from build123d import *

# Parameters (mm, degrees)
F1_DEPTH = 3
F2_DEPTH = 150
F3_R     = 30.5
F3_R_2   = 1
F4_DEPTH = 5
F5_R     = 30.5
F5_R_2   = 1
F6_DEPTH = 5


with BuildPart() as f1:
    # F0 (on Top) → F1 (new body)
    with BuildSketch(Plane.XY):
        Polygon((-91.6025403784, 38.2228657698), (-91.6025403784, -34.6638855762), (-1.3397459622, -86.7771342302), (105, -86.7771342302), (105, 38.2228657698), align=None)
        Polygon((100, -81.7771342302), (0, -81.7771342302), (-86.6025403784, -31.7771342302), (-86.6025403784, 33.2228657698), (100, 33.2228657698), align=None, mode=Mode.SUBTRACT)
        Polygon((-86.6025403784, -31.7771342302), (0, -81.7771342302), (100, -81.7771342302), (100, 33.2228657698), (-86.6025403784, 33.2228657698), align=None)
    extrude(amount=F1_DEPTH)

    # F0 (on Top) → F2 (join)
    with BuildSketch(Plane.XY):
        Polygon((-91.6025403784, 38.2228657698), (-91.6025403784, -34.6638855762), (-1.3397459622, -86.7771342302), (105, -86.7771342302), (105, 38.2228657698), align=None)
        Polygon((100, -81.7771342302), (0, -81.7771342302), (-86.6025403784, -31.7771342302), (-86.6025403784, 33.2228657698), (100, 33.2228657698), align=None, mode=Mode.SUBTRACT)
    extrude(amount=F2_DEPTH)

    # F3 (on face) → F4 (cut)
    with BuildSketch(Plane.XZ.offset(86.7771342302)):
        with Locations((51.8301270189, 39.6802276373)):
            Circle(F3_R)
        with Locations((25.3301270189, 13.1802276373)):
            Circle(F3_R_2)
        with Locations((78.3301270189, 13.1802276373)):
            Circle(F3_R_2)
        with Locations((78.3301270189, 66.1802276373)):
            Circle(F3_R_2)
        with Locations((25.3301270189, 66.1802276373)):
            Circle(F3_R_2)
    extrude(amount=-F4_DEPTH, mode=Mode.SUBTRACT)

    # F5 (on face) → F6 (cut)
    with BuildSketch(Plane(origin=(-37.910537846, -65.6629776916, 0), x_dir=(0.8660254038, -0.5, 0), z_dir=(-0.5, -0.8660254038, 0))):
        with Locations((-10.3275869042, 39.1066893935)):
            Circle(F5_R)
        with Locations((16.1724130958, 65.6066893935)):
            Circle(F5_R_2)
        with Locations((16.1724130958, 12.6066893935)):
            Circle(F5_R_2)
        with Locations((-36.8275869042, 65.6066893935)):
            Circle(F5_R_2)
        with Locations((-36.8275869042, 12.6066893935)):
            Circle(F5_R_2)
    extrude(amount=-F6_DEPTH, mode=Mode.SUBTRACT)


solid = f1.part
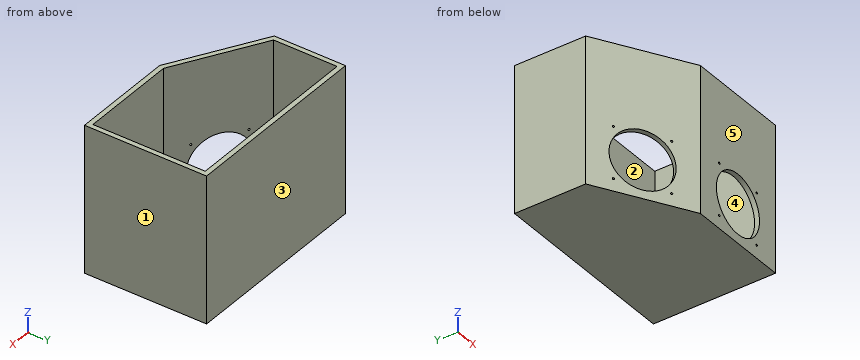
Read the model definition and answer for the solid it produces. Units are mm, in the model's axes. Face numbers are marked on the shaded views. A direction names the side the tool comes from. Coordinates: 2 decimals unless noted, no trailing zeros. Write each loop counter-clockwise with the first axis right and the second up, starting at its lowest first coordinate (ties: lowest second). Pieces come first, ordered by that corner, then holes. Notation, with made-up numbers: (69, 2) -> (110, 2) arc R23 cw to (110, 19) -> close; hole circle Ø9 at (-29.5, 61). An arc over 180 degrees is marked (long way). Return JSON: item names as keys, results as strings.
(1) The part is cut by section D-D on x = 88. Give the vertices of the cut face in (y, z).
Answers below:
{"outline": "(-86.78, 0) -> (38.22, 0) -> (38.22, 150) -> (33.22, 150) -> (33.22, 3) -> (-81.78, 3) -> (-81.78, 150) -> (-86.78, 150) -> close"}
(2) The part is cut by section B-B on z = 74.5. Give the vertices of the cut face in (x, y).
Answers below:
{"outline": "(-91.6, -34.66) -> (-1.34, -86.78) -> (105, -86.78) -> (105, 38.22) -> (-91.6, 38.22) -> close; hole (-86.6, -31.78) -> (0, -81.78) -> (100, -81.78) -> (100, 33.22) -> (-86.6, 33.22) -> close"}
(3) The part is cut by section C-C on y = -17.5. Give the vertices of the cut face in (x, z).
Answers below:
{"outline": "(-91.6, 0) -> (105, 0) -> (105, 150) -> (100, 150) -> (100, 3) -> (-86.6, 3) -> (-86.6, 150) -> (-91.6, 150) -> close"}
(4) Consider line 1 along X through (y, z) = (20, 10.5); line 2 along Y through (x, z) = (14, 20); line 3 along Z through (x, y) = (86, 3). Determine where each line is inside the solid, lowest interval first. Write a range as from..to.
Answers below:
{"line 1": "-91.6..-86.6, 100..105", "line 2": "-86.78..-81.78, 33.22..38.22", "line 3": "0..3"}
(5) For a pull along X with two mould halves and no side action, classify the marked faces 1, 2 and 3 as pulls with the +X half, pulls with the -X half, needs draft (parallel to the pull), parting line crosses it, or undercut.
Answers below:
{"face 1": "pulls with the +X half", "face 2": "undercut", "face 3": "needs draft"}
(6) The part is cut by section A-A on x = 30. Give the vertices of the cut face in (y, z), then the cut area to 3 significant figures.
Answers below:
{"outline": "(-86.78, 0) -> (38.22, 0) -> (38.22, 150) -> (33.22, 150) -> (33.22, 3) -> (-81.78, 3) -> (-81.78, 18.38) -> (-86.78, 18.38) -> close; (-86.78, 60.98) -> (-81.78, 60.98) -> (-81.78, 150) -> (-86.78, 150) -> close", "area": "1,630 mm^2"}
(7) Each of these flat-tipped pins is pushed along its axis until it touches: P1, Ø4, axis at x = -10, z = 27.5, coming from the -Y side; P2, Ø3, axis at x = 38.5, y = -9.5, coming from the +Z side. Where does it stop, or does it pass through?
Answers below:
{"P1": "y = -82.93", "P2": "z = 3"}
(8) Which of the six approach directions +Z, -Z, +X, -X, +Y, -Y give full straight-line access (tool end or side, diameter ignored) to the marked faces 4 and 5?
Answers below:
{"face 4": "+Z", "face 5": "+Z, -Z, +X, -X, -Y"}
